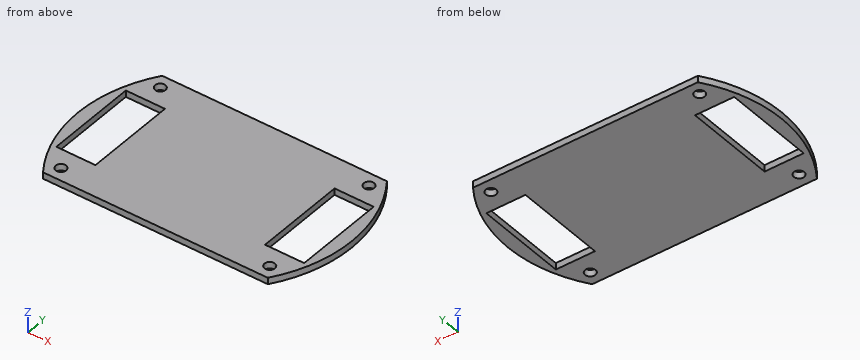
from build123d import *

# Parameters (mm, degrees)
ESQUISSE1_R             = 105
ESQUISSE1_R_2           = 4
ESQUISSE1_W             = 30
ESQUISSE1_H             = 70
BOSS_EXTRU_1_DEPTH      = 5
ESQUISSE2_W             = 250
ESQUISSE2_H             = 50
ENL_V_MAT_EXTRU_1_DEPTH = 149.576579581


with BuildPart() as part:
    # Esquisse1 → Boss.-Extru.1 (new body)
    with BuildSketch(Plane.XY):
        Circle(ESQUISSE1_R)
        with Locations((-80, 50)):
            Circle(ESQUISSE1_R_2, mode=Mode.SUBTRACT)
        with Locations(Location((80, 50, 0), (0, 0, 180))):
            Circle(ESQUISSE1_R_2, mode=Mode.SUBTRACT)
        with Locations((80, -50)):
            Circle(ESQUISSE1_R_2, mode=Mode.SUBTRACT)
        with Locations(Location((-80, -50, 0), (0, 0, 180))):
            Circle(ESQUISSE1_R_2, mode=Mode.SUBTRACT)
        with Locations((-80, 0)):
            Rectangle(ESQUISSE1_W, ESQUISSE1_H, mode=Mode.SUBTRACT)
        with Locations((80, 0)):
            Rectangle(ESQUISSE1_W, ESQUISSE1_H, mode=Mode.SUBTRACT)
    extrude(amount=BOSS_EXTRU_1_DEPTH)

    # Esquisse2 → Enlèv. mat.-Extru.1 (cut, through all)
    with BuildSketch(Plane.XY.offset(5)):
        with Locations((0, 85)):
            Rectangle(ESQUISSE2_W, ESQUISSE2_H)
        with Locations((0, -85)):
            Rectangle(ESQUISSE2_W, ESQUISSE2_H)
    extrude(amount=-ENL_V_MAT_EXTRU_1_DEPTH, mode=Mode.SUBTRACT)


solid = part.part
Geometry: final body of the model. Coordinates: model frame, mm. Coordinates: 2 decimals unless noted, no trailing zeros. Loops run counter-clockwise (first coordinate to the right, second up) from the corner with the lowest first, then second, coordinate; pieces in that order, holes last. Notation, with made-up numbers: M 52.5,29 L 56.5,29 A26 ccw 56.5,43 Z; hole C 83,35.5 d6. An arc over 180 degrees is marked long. One line per item, written item: value. Start each with the question number.
1) Cut plane C-C (y = 16). Return loops of the section in (x, z), then the cut area to 3 significant figures.
2) Cut plane D-D (y = -33). Return loops of the section in (x, z), then the cut area to 3 significant figures.
3) Cut plane A-A (x = -80). Return loops of the section in (y, z).
4) Cut plane B-B (z = 2.2). Return loops of the section in (x, y), then the cut area to 3 significant figures.
5) Pin query (flat end, axial travel): P1, Ø1.5, axis at y = -40, z = 3, coming from the -X side; P2, Ø3, axis at y = -22, z = 1, coming from the +X side; P3, Ø1.5, axis at y = 13, z = 3.5, coming from the -X side. Return the tip coordinate at first contact, or that it passes through.
6) Material intervals for L1, parallel to Y at x = 80, z = 3.25; L2, parallel to Y at x = 70, z = 4.15; L3, parallel to X at y = 8, z = 2.3, sorted ascending. Write a range as from..to.
Evaluation:
1. outline: M -103.77,0 L -95,0 L -95,5 L -103.77,5 Z; M -65,0 L 65,0 L 65,5 L -65,5 Z; M 95,0 L 103.77,0 L 103.77,5 L 95,5 Z
1. area: 738 mm^2
2. outline: M -99.68,0 L -95,0 L -95,5 L -99.68,5 Z; M -65,0 L 65,0 L 65,5 L -65,5 Z; M 95,0 L 99.68,0 L 99.68,5 L 95,5 Z
2. area: 697 mm^2
3. outline: M -60,0 L -54,0 L -54,5 L -60,5 Z; M -46,0 L -35,0 L -35,5 L -46,5 Z; M 35,0 L 46,0 L 46,5 L 35,5 Z; M 54,0 L 60,0 L 60,5 L 54,5 Z
4. outline: M -86.17,-60 L 86.17,-60 A105 ccw 86.17,60 L -86.17,60 A105 ccw Z; hole M -95,-35 L -65,-35 L -65,35 L -95,35 Z; hole C -80,-50 d8; hole C -80,50 d8; hole M 65,-35 L 95,-35 L 95,35 L 65,35 Z; hole C 80,-50 d8; hole C 80,50 d8
4. area: 19,400 mm^2
5. P1: x = -97.39
5. P2: x = 102.98
5. P3: x = -104.28
6. L1: -60..-54, -46..-35, 35..46, 54..60
6. L2: -60..-35, 35..60
6. L3: -104.69..-95, -65..65, 95..104.69
